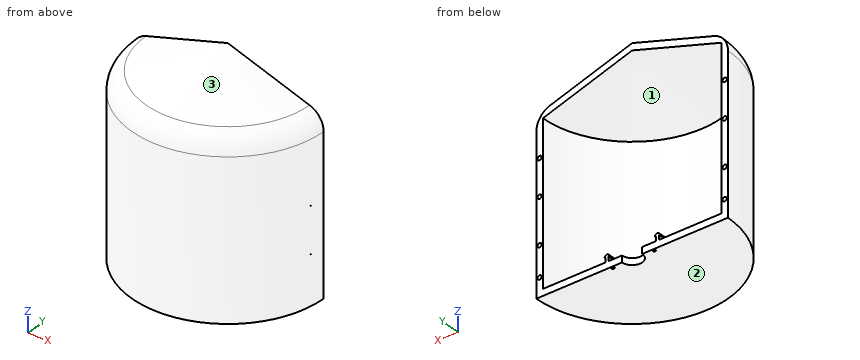
```python
from build123d import *

# Parameters (mm, degrees)
REVOLVE1_ANGLE           = 180
BOSS_EXTRUDE8_REACH      = 185.507
BOSS_EXTRUDE8_END_RADIUS = 88.5
SKETCH7_R                = 10
SKETCH7_R_2              = 1.5
CUT_EXTRUDE1_DEPTH       = 10
SKETCH3_R                = 2.075
CUT_EXTRUDE3_DEPTH       = 15
FILLET1_R                = 20


with BuildPart() as part:
    # Sketch1 → Revolve1 (revolve)
    with BuildSketch(Plane(origin=(0, 0, 0), x_dir=(1, 0, 0), z_dir=(0, 1, 0))):
        Polygon((0, 75), (95, 75), (95, -95), (0, -125), align=None)
    revolve(axis=Axis((0, 0, 125), (0, 0, -1)), revolution_arc=REVOLVE1_ANGLE)

    # Sketch2 → Cut-Revolve3 (revolve, cut)
    with BuildSketch(Plane(origin=(0, 0, 0), x_dir=(1, 0, 0), z_dir=(0, 1, 0))):
        Polygon((0, 68.5), (0, -118.183600921), (88.5, -90.2362325), (88.5, 68.5), align=None)
    revolve(axis=Axis((0, 0, -68.5), (0, 0, 1)), mode=Mode.SUBTRACT)

    # Boss-Extrude8: up to this cylinder (the profile starts inside it)
    boss_extrude8_end = Plane(origin=(0, 0, -64.938407), z_dir=(0, 0, -1)) * Cylinder(BOSS_EXTRUDE8_END_RADIUS, 549.014, mode=Mode.PRIVATE)
    # Sketch5 → Boss-Extrude8 (add, up to the surface)
    with BuildSketch(Plane(origin=(0, 0, 0), x_dir=(1, 0, 0), z_dir=(0, 1, 0)), mode=Mode.PRIVATE) as boss_extrude8_sk1:
        with BuildLine():
            Line((23.5, 64), (23.5, 68.5))
            Line((23.5, 68.5), (26.5, 68.5))
            Line((26.5, 68.5), (26.5, 64))
            Line((26.5, 64), (27.4, 64))
            ThreePointArc((27.4, 64), (25, 61.6), (22.6, 64))
            Line((22.6, 64), (23.5, 64))
        make_face()
    boss_extrude8_tool1 = extrude(boss_extrude8_sk1.sketch, amount=-BOSS_EXTRUDE8_REACH, mode=Mode.PRIVATE) & boss_extrude8_end
    add(boss_extrude8_tool1.solids().sort_by_distance((25, 0, -64.938407))[0])
    # Sketch5 → Boss-Extrude8 (add, up to the surface)
    with BuildSketch(Plane(origin=(0, 0, 0), x_dir=(1, 0, 0), z_dir=(0, 1, 0)), mode=Mode.PRIVATE) as boss_extrude8_sk2:
        with BuildLine():
            Line((-27.4, 64), (-26.5, 64))
            Line((-26.5, 64), (-26.5, 68.5))
            Line((-26.5, 68.5), (-23.5, 68.5))
            Line((-23.5, 68.5), (-23.5, 64))
            Line((-23.5, 64), (-22.6, 64))
            ThreePointArc((-22.6, 64), (-25, 61.6), (-27.4, 64))
        make_face()
    boss_extrude8_tool2 = extrude(boss_extrude8_sk2.sketch, amount=-BOSS_EXTRUDE8_REACH, mode=Mode.PRIVATE) & boss_extrude8_end
    add(boss_extrude8_tool2.solids().sort_by_distance((-25, 0, -64.938407))[0])

    # Sketch7 → Cut-Extrude1 (cut)
    with BuildSketch(Plane.XY.offset(-68.5)):
        Circle(SKETCH7_R)
        with Locations((20.425168298, -1.75)):
            Circle(SKETCH7_R_2)
        with Locations(Location((-20.425168298, -1.75, 0), (0, 0, 180))):
            Circle(SKETCH7_R_2)
    extrude(amount=-CUT_EXTRUDE1_DEPTH, mode=Mode.SUBTRACT)

    # Sketch3 → Cut-Extrude3 (cut)
    with BuildSketch(Plane(origin=(0, 0, 0), x_dir=(1, 0, 0), z_dir=(0, 1, 0))):
        with Locations(Location((-91.75, 56.5, 0), (0, 0, 180))):
            Circle(SKETCH3_R)
        with Locations(Location((-91.75, 26.5, 0), (0, 0, 180))):
            Circle(SKETCH3_R)
        with Locations(Location((-91.75, -18.5, 0), (0, 0, 180))):
            Circle(SKETCH3_R)
        with Locations(Location((-91.75, -54.5, 0), (0, 0, 180))):
            Circle(SKETCH3_R)
        with Locations(Location((91.75, -54.5, 0), (0, 0, 7.270772685))):
            Circle(SKETCH3_R)
        with Locations(Location((91.75, -18.5, 0), (0, 0, 7.270772685))):
            Circle(SKETCH3_R)
        with Locations(Location((91.75, 26.5, 0), (0, 0, 7.270772685))):
            Circle(SKETCH3_R)
        with Locations(Location((91.75, 56.5, 0), (0, 0, 7.270772685))):
            Circle(SKETCH3_R)
    extrude(amount=-CUT_EXTRUDE3_DEPTH, mode=Mode.SUBTRACT)

    # Fillet1
    fillet1_edges = [part.edges().sort_by_distance(p)[0] for p in [
        (0, -95, 95),
    ]]
    fillet(fillet1_edges, radius=FILLET1_R)


solid = part.part
```
Model file for the job. Use its own axes, mm. Face numbers are marked on the shaded views. Coordinates: 2 decimals unless noted, no trailing zeros. Loops run counter-clockwise (first coordinate to the right, second up) from the corner with the lowest first, then second, coordinate; pieces in that order, holes last. Notation, with made-up numbers: M 10,-29.5 L 60,-29.5 A29 ccw 60,0.5 Z; hole C 49,22 d5. An arc over 180 degrees is marked long. Use CSV: the item, a comma, the result in double quotes. Start each with the question number.
1. Probe probe 1 along X at (y, z) = (-7.75, 54.5) (3 decimals); probe 2 along Z at (x, y) = (-91, -5); probe 3 along X at (y, z) = (-5.75, -26.5) (3 decimals). List the from-to ranges inside material, lowest first. Write a range as [from, to].
2. Flat gauge pins, fed straight in: pin 1 (3.5 mm diameter, centred on x = -91.75, z = 18.5, fed in from +Y); pin 2 (1 mm diameter, centred on y = -40, z = 31, fed in from -X); pin 3 (2 mm diameter, centred on y = -28.5, z = -66, fed in from +X). Where does each tip first touch, or does it go through?
3. Two-plate mould, pull along X, no slides. Class the marked faces 1, 2 and 3: pulls with the +X half, pulls with the -X half, needs draft (parallel to the pull), parting line crosses it, or undercut.
4. Band-saw the part on A-A, the plane z = 70.5. List the corners of the cut face in (x, y), then the cut area to 3 significant figures.
Entries:
1,probe 1,"x = [-94.683, -93.825], [-89.675, -88.16], [88.16, 89.675], [93.825, 94.683]"
1,probe 2,"z = [-75, -58.43], [-54.57, -28.43], [-24.57, 16.57], [20.43, 52.57], [56.43, 92.16]"
1,probe 3,"x = [-94.826, -93.825], [-89.675, -88.313], [88.313, 89.675], [93.825, 94.826]"
2,pin 1,"stops at y = -15"
2,pin 2,"stops at x = -86.4"
2,pin 3,"stops at x = 90.93"
3,face 1,"undercut"
3,face 2,"needs draft"
3,face 3,"parting line crosses it"
4,outline,"M -95,0 A95 ccw 95,0 L 88.5,0 A88.5 cw -88.5,0 Z"
4,area,"1,870 mm2"
